Check sheet for the drawn part. Datum: minimum x, y, z corner. Units: mm. A direction names the side the tool comes from. Give positions to 0.01 mm unless a question says otherwise; leave off trailing zeros. Write each loop counter-clockwise with the first axis right and the second up, starting at its lowest first coordinate (ties: lowest second). Pieces come first, ordered by that corner, then holes. Notation, with made-up numbers: M -36,63.5 L 21,63.5 A23 ccw 21,90.5 Z; hole C 77,75 d11. An arc over 180 degrees is marked long. Use CSV: the item, a comma, the result in double quotes. Start each with the question number.
1. Cross-section at C-C, the plane y = 0.5. Enter the section's corners in (x, z).
2. Scan lines: line 1 (Y direction, x = 17, z = 12.25); line 2 (Z direction, x = 17.25, y = 4); line 3 (X direction, y = 6.75, z = 15). Record each from-to range of solid material in increasing order.
3. Cross-section at B-B, the plane x = 16. Enter the section's corners in (y, z), and give its area (3 significant figures).
4. Depth check by flat-ended pin: P1, Ø1, axis at x = 6, y = 3.5, coming from the -Z side; P2, Ø1.2, axis at y = 6, z = 16.5, coming from the -X side. Enter the tip coordinate at first touch or a pass-through.
5. Access from +Z, -Z, +X, -X, +Y, -Y to the whole of each face (thin tool, end or side, straight path). Record for the marked faces 4 and 5.
6. Cross-section at A-A, the plane z = 14.75. Enter the section's corners in (x, y).
7. Mould release check, pull along Y, two halves, no side actions. Record for the marked faces 1, 2 and 3: +Y half, -Y half, draft (parallel to the pull), parting line (faces both ways), or undercut.
8. Cross-section at D-D, the plane y = 5. Enter the section's corners in (x, z).
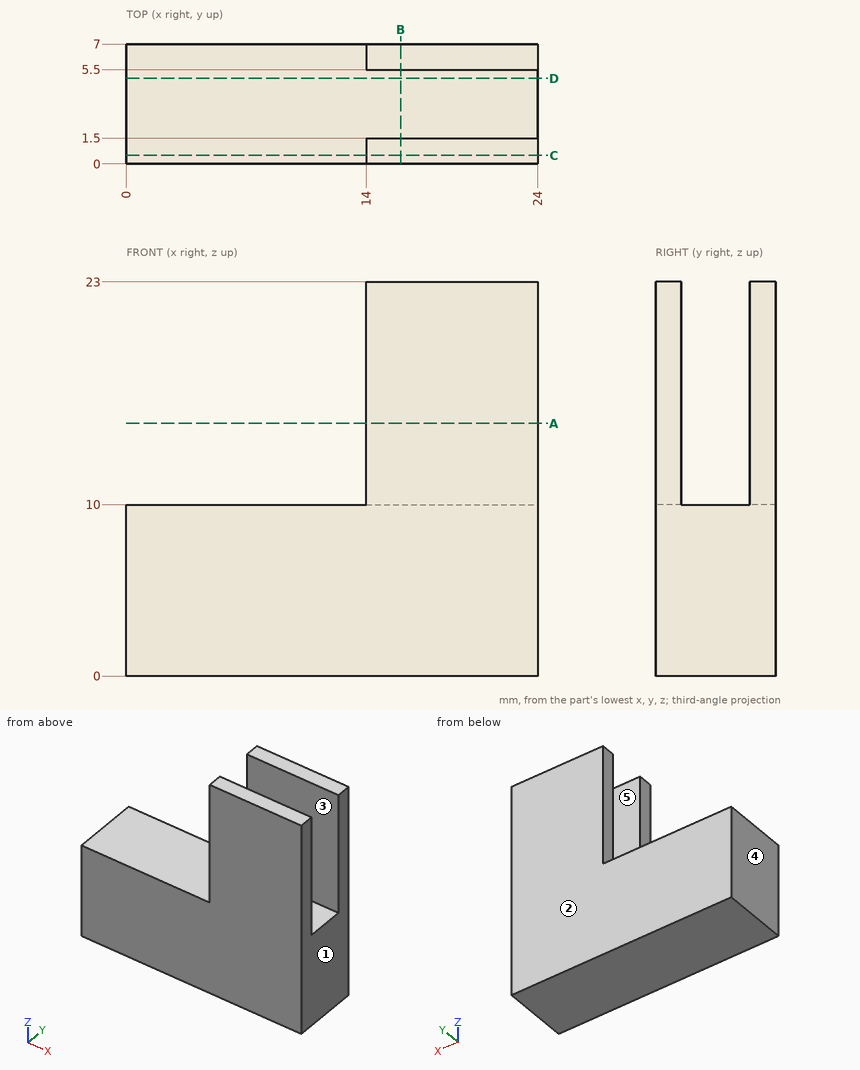
Worked answers:
1,outline,"M 0,0 L 24,0 L 24,23 L 14,23 L 14,10 L 0,10 Z"
2,line 1,"y = 0 to 1.5, 5.5 to 7"
2,line 2,"z = 0 to 10"
2,line 3,"x = 14 to 24"
3,outline,"M 0,0 L 7,0 L 7,23 L 5.5,23 L 5.5,10 L 1.5,10 L 1.5,23 L 0,23 Z"
3,area,"109 mm^2"
4,P1,"stops at z = 0"
4,P2,"stops at x = 14"
5,face 4,"+Z, -Z, -X, +Y, -Y"
5,face 5,"+Z, +X, -X"
6,outline,"M 14,0 L 24,0 L 24,1.5 L 14,1.5 Z; M 14,5.5 L 24,5.5 L 24,7 L 14,7 Z"
7,face 1,"draft"
7,face 2,"+Y half"
7,face 3,"undercut"
8,outline,"M 0,0 L 24,0 L 24,10 L 0,10 Z"
